Autodesk Inventor part; units mm, degrees
ref_plane "YZ Plane" through (0, 0, 0) normal (1, 0, 0) x (0, 1, 0)
ref_plane "XZ Plane" through (0, 0, 0) normal (0, 1, 0) x (-1, 0, 0)
ref_plane "XY Plane" through (0, 0, 0) normal (0, 0, 1) x (1, 0, 0)
sketch "Sketch1" plane through (0, 0, 0) normal (1, 0, 0) x (0, 1, 0)
  circle A0 centre (0, 0) radius 6
  dimension "hubouter" = 12
extrude "Extrusion1" add sketch "Sketch1" along normal blind 6
sketch "Sketch2" plane through (0, 0, 0) normal (-1, 0, 0) x (0, 0, 1)
  circle A0 centre (0, 0) radius 1.5
  dimension "hole" = 3
hole "Hole1" at (0, 0, 0) direction (1, 0, 0) diameter 5.5 end through all
sketch "Sketch3" plane through (0, 0, 0) normal (-1, 0, 0) x (0, 0, 1)
  circle A0 centre (0, 0) radius 16.5
  circle A1 centre (0, 0) radius 25
  circle A2 centre (0, 0) radius 6
  line L0 (6, 0) -> (26, 0)
  line L1 (16.1025, -3.6) -> (4.8, -3.6)
  line L2 (16.1025, 3.6) -> (4.8, 3.6)
  arc A3 (4.8, -3.6) -> (4.8, 3.6) centre (0, 0) ccw
  dimension "innerdiam" = 33
  dimension "outerdiam" = 50
extrude "Extrusion2" add sketch "Sketch3" against normal blind 20
sketch "Sketch5" plane through (0, 0, 0) normal (1, 0, 0) x (0, 1, 0)
  circle A0 centre (0, 0) radius 6 construction
  line L0 (0, 6) -> (22.3607, 6)
  circle A1 centre (0, 0) radius 2.75
  line L1 (0, -6) -> (23.0083, -2.5724)
  line L2 (23.0083, -2.5724) -> (22.7003, -2.6183)
  arc A2 (0, -6) -> (0, 6) centre (0, 0) ccw
  arc A3 (23.0083, -2.5724) -> (22.3607, 6) centre (0, 0) ccw
  point P0 (1.7489, -5.7395)
extrude "Extrusion4" add sketch "Sketch5" along normal blind 3 contours L0 A3 L1 A2
pattern_circular "Circular Pattern2" count 3 over 360 about axis through (-10, 0, 0) along (1, 0, 0) of "Extrusion4"
ref_plane "Work Plane4" through (3, 16.1022, -3.6012) normal (1, 0, 0) x (0, 1, 0)
properties part number "Reaction_wheel_dr - Copy (3.3)" material "Steel, Carbon"
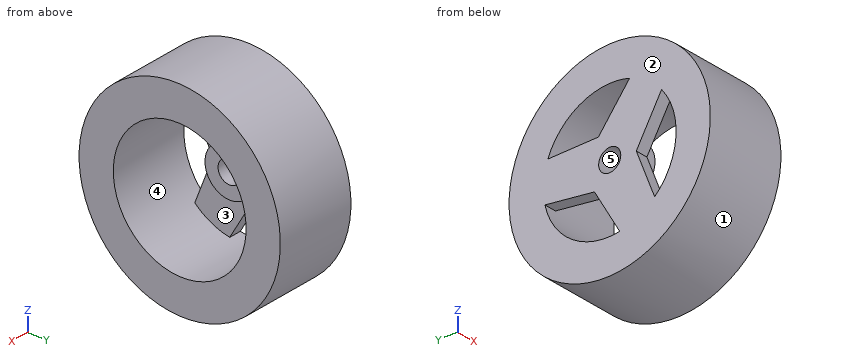
Work out the finished part from the listing and answer in its coordinate system (mm). Face numbers are marked on the shaded views. A direction names the side the tool comes from. Coordinates: 2 decimals unless noted, no trailing zeros. Loops run counter-clockwise (first coordinate to the right, second up) from the corner with the lowest first, then second, coordinate; pieces in that order, holes last. Notation, with made-up numbers: (84.25, 12) - (122.25, 12) arc R22 cw to (122.25, 32) - close; hole circle Ø5 at (-8, -1.5). An arc over 180 degrees is marked (long way). Use a Markdown table: item, result.
Item 1: Consider probe 1 along Y at (x, z) = (4.75, 0); probe 2 along Y at (x, z) = (2.6, 0); probe 3 along Y at (x, z) = (9.25, 0). Determine where each line is inside the solid, lowest interval first. Write a range as from..to.
Evaluation:
| item | result |
|---|---|
| probe 1 | y = -25..-16.5, -6..-2.75, 2.75..6, 16.5..25 |
| probe 2 | y = -25..-16.5, -6.93..-2.75, 2.75..25 |
| probe 3 | y = -25..-16.5, 16.5..25 |
Item 2: Given pin 1 Ø2 at (x, y) = (9, 19.5) entering from -Z; pin 2 Ø8 at (y, z) = (4, 8) entering from +X; pin 3 Ø6 at (x, y) = (11.5, -4.5) entering from +Z; pin 4 Ø4.5 at (y, z) = (0, 0) entering from -X, each flat-ended and moving along its own axis, determine where each tip first touches the part or whether it passes through.
Evaluation:
| item | result |
|---|---|
| pin 1 | stops at z = -16.82 |
| pin 2 | stops at x = 6 |
| pin 3 | stops at z = 24.95 |
| pin 4 | passes through |
Item 3: Find section B-B, the plane z = 11.5. Determine the outline of the cut face in (x, y).
Evaluation:
| item | result |
|---|---|
| outline | (0, -22.2) - (20, -22.2) - (20, -11.83) - (3, -11.83) - (3, -1.56) - (0, -1.56) - close; (0, 11.83) - (20, 11.83) - (20, 22.2) - (0, 22.2) - close |
Item 4: Find section D-D, the plane z = -11.5. Determine the outline of the cut face in (x, y), and give its area (3 significant figures).
Evaluation:
| item | result |
|---|---|
| outline | (0, -22.2) - (20, -22.2) - (20, -11.83) - (0, -11.83) - close; (0, -10.92) - (3, -10.92) - (3, 0.29) - (0, 0.29) - close; (0, 11.83) - (20, 11.83) - (20, 22.2) - (0, 22.2) - close |
| area | 448 mm2 |
Item 5: Find section C-C, the plane y = 14.5. Determine the outline of the cut face in (x, z), and give its area (3 significant figures).
Evaluation:
| item | result |
|---|---|
| outline | (0, -20.37) - (20, -20.37) - (20, -7.87) - (0, -7.87) - close; (0, -3.84) - (3, -3.84) - (3, 6) - (0, 6) - close; (0, 7.87) - (20, 7.87) - (20, 20.37) - (0, 20.37) - close |
| area | 529 mm2 |
Item 6: For the marked faces 4 and 5, determine the directions among +Z, -Z, +X, -X, +Y, -Y from which every point of the face is accessible in a straight line to the end or side of a thin tool.
Evaluation:
| item | result |
|---|---|
| face 4 | +X |
| face 5 | +X, -X |
Item 7: Find section A-A, the plane y = -14.5. Determine the outline of the cut face in (x, z).
Evaluation:
| item | result |
|---|---|
| outline | (0, -20.37) - (20, -20.37) - (20, -7.87) - (0, -7.87) - close; (0, 7.87) - (20, 7.87) - (20, 20.37) - (0, 20.37) - close |
Item 8: The mould has two halves that part along Y. Classify the marked faces 1, 2 and 3: +Y half, -Y half, draft (parallel to the pull), parting line (faces both ways), or undercut.
Evaluation:
| item | result |
|---|---|
| face 1 | parting line |
| face 2 | draft |
| face 3 | undercut |
